Could you check a few things on this model? Use its own coordinates, in mm. A direction names the side the tool comes from. Round coordinates to 2 decimals unless told otherwise and drop trailing zeros. Loops run counter-clockwise (first coordinate to the right, second up) from the corner with the lowest first, then second, coordinate; pieces in that order, holes last.
from build123d import *
from build123d.topology import SkipClean

# Parameters (mm, degrees)
BOSS_EXTRUDE1_DEPTH         = 31.75
BOSS_EXTRUDE4_DEPTH         = 38.1
SKETCH11_R                  = 12.7
BOSS_EXTRUDE5_DEPTH         = 19.05
F_1_4_20_TAPPED_HOLE3_D     = 5.1054
F_1_4_20_TAPPED_HOLE3_DEPTH = 38.1
F_1_4_20_TAPPED_HOLE3_TIP   = 1.533816902
F_1_4_20_TAPPED_HOLE4_D     = 5.1054
F_1_4_20_TAPPED_HOLE4_DEPTH = 11.43
F_1_4_20_TAPPED_HOLE4_TIP   = 1.533816902
CUT_EXTRUDE3_DEPTH          = 3.175
SKETCH17_R                  = 15.875
CUT_EXTRUDE4_DEPTH          = 15.875
FILLET3_R                   = 1.5875
CUT_EXTRUDE5_DEPTH          = 6.35
FILLET4_R                   = 1.5875


with BuildPart() as part:
    # Sketch1 → Boss-Extrude1 (new body)
    with BuildSketch(Plane.XY):
        with BuildLine():
            Line((18.072416828, 26.104602085), (30.120694713, -10.040231571))
            Line((30.120694713, -10.040231571), (6.024138943, -18.072416828))
            ThreePointArc((6.024138943, -18.072416828), (-18.072416828, -6.024138943), (-6.024138943, 18.072416828))
            Line((-6.024138943, 18.072416828), (18.072416828, 26.104602085))
        make_face()
    extrude(amount=BOSS_EXTRUDE1_DEPTH)

    # Sketch10 → Boss-Extrude4 (add)
    with BuildSketch(Plane(origin=(-6.024138943, 18.072416828, 0), x_dir=(0.9486832980505138, 0.31622776601683816, 0), z_dir=(-0.31622776601683816, 0.9486832980505138, 0))):
        Polygon((25.4, 0), (31.75, 0), (40.015050599, -37.192726958), (27.240344607, -40.031550568), (25.4, -31.75), align=None)
    extrude(amount=-BOSS_EXTRUDE4_DEPTH)

    # Sketch11 → Boss-Extrude5 (add)
    with BuildSketch(Plane.XY.offset(31.75)):
        with Locations(Location((0, 0, 0), (0, 0, 180))):
            Circle(SKETCH11_R)
    extrude(amount=BOSS_EXTRUDE5_DEPTH)

    # 1/4-20 Tapped Hole3
    with Locations(Plane.XY.offset(50.8)):
        with Locations((0, 0)):
            Hole(F_1_4_20_TAPPED_HOLE3_D / 2, depth=F_1_4_20_TAPPED_HOLE3_DEPTH)
            with Locations((0, 0, -(F_1_4_20_TAPPED_HOLE3_DEPTH + F_1_4_20_TAPPED_HOLE3_TIP / 2))):  # 118° drill point
                Cone(0, F_1_4_20_TAPPED_HOLE3_D / 2, F_1_4_20_TAPPED_HOLE3_TIP, mode=Mode.SUBTRACT)

    # 1/4-20 Tapped Hole4
    with Locations(Plane(origin=(28.703250202, 9.567750067, -6.723529533), x_dir=(-0.2057983060639255, -0.06859943535464187, -0.9761870592720655), z_dir=(0.9260923589044555, 0.30869745296815215, -0.21693046192214882))):
        with Locations((-38.637542166, 12.7), (-16.412542166, 6.35), (-16.412542166, -6.35), (-38.637542166, -12.7)):
            Hole(F_1_4_20_TAPPED_HOLE4_D / 2, depth=F_1_4_20_TAPPED_HOLE4_DEPTH)
            with Locations((0, 0, -(F_1_4_20_TAPPED_HOLE4_DEPTH + F_1_4_20_TAPPED_HOLE4_TIP / 2))):  # 118° drill point
                Cone(0, F_1_4_20_TAPPED_HOLE4_D / 2, F_1_4_20_TAPPED_HOLE4_TIP, mode=Mode.SUBTRACT)

    # Sketch16 → Cut-Extrude3 (cut)
    with BuildSketch(Plane(origin=(0, 0, 0), x_dir=(-1, 0, 0), z_dir=(0, 0, -1))):
        with BuildLine():
            Line((-30.578183366, -6.540991497), (-16.999386581, -3.994967099))
            ThreePointArc((-16.999386581, -3.994967099), (-15.110000404, -8.753673173), (-11.921633961, -12.759841298))
            Line((-11.921633961, -12.759841298), (-30.578183366, -6.540991497))
        make_face()
        with BuildLine():
            Line((-31.84160072, -5.162718019), (-17.29194463, -2.434657503))
            ThreePointArc((-17.29194463, -2.434657503), (-16.566382092, 5.522127364), (-12.372761203, 12.32289278))
            Line((-12.372761203, 12.32289278), (-22.375649764, 23.235134847))
            Line((-22.375649764, 23.235134847), (-31.84160072, -5.162718019))
        make_face()
        with BuildLine():
            Line((-1.88140239, 17.360853415), (-20.537951794, 23.579703217))
            Line((-20.537951794, 23.579703217), (-11.202529005, 13.395605628))
            ThreePointArc((-11.202529005, 13.395605628), (-6.83579642, 16.068938781), (-1.88140239, 17.360853415))
        make_face()
    extrude(amount=-CUT_EXTRUDE3_DEPTH, mode=Mode.SUBTRACT)

    # Sketch17 → Cut-Extrude4 (cut)
    with BuildSketch(Plane(origin=(0, 0, 0), x_dir=(-1, 0, 0), z_dir=(0, 0, -1))):
        Circle(SKETCH17_R)
    extrude(amount=-CUT_EXTRUDE4_DEPTH, mode=Mode.SUBTRACT)

    # Fillet3
    fillet3_edges = [part.edges().sort_by_distance(p)[0] for p in [
        (31.84160072, -5.162718019, 1.5875),
        (22.375649764, 23.235134847, 1.5875),
        (12.372761203, 12.32289278, 1.5875),
        (17.29194463, -2.434657503, 1.5875),
        (11.202529005, 13.395605628, 1.5875),
        (20.537951794, 23.579703217, 1.5875),
        (1.88140239, 17.360853415, 1.5875),
        (16.999386581, -3.994967099, 1.5875),
        (11.921633961, -12.759841298, 1.5875),
        (30.578183366, -6.540991497, 1.5875),
    ]]
    fillet(fillet3_edges, radius=FILLET3_R)

    # Sketch19 → Cut-Extrude5 (cut)
    with SkipClean():  # the faces are left unmerged after this step: merging them gives an invalid solid
        with BuildSketch(Plane(origin=(0, 0, 15.875), x_dir=(-1, 0, 0), z_dir=(0, 0, -1))):
            with BuildLine():
                Line((1.5875, 4.490128061), (1.5875, 15.795425564))
                ThreePointArc((1.5875, 15.795425564), (9.33109088, 12.843144786), (14.531777932, 6.390857152))
                Line((14.531777932, 6.390857152), (3.779801072, 2.897328097))
                ThreePointArc((3.779801072, 2.897328097), (2.799327264, 3.852943436), (1.5875, 4.490128061))
            make_face()
            with BuildLine():
                Line((-1.5875, 4.490128061), (-1.5875, 15.795425564))
                ThreePointArc((-1.5875, 15.795425564), (-9.33109088, 12.843144786), (-14.531777932, 6.390857152))
                Line((-14.531777932, 6.390857152), (-3.779801072, 2.897328097))
                ThreePointArc((-3.779801072, 2.897328097), (-2.799327264, 3.852943436), (-1.5875, 4.490128061))
            make_face()
            with BuildLine():
                Line((4.76093003, -0.122276342), (15.512906889, 3.371252713))
                ThreePointArc((15.512906889, 3.371252713), (15.098022196, -4.905644786), (10.568632679, -11.845658627))
                Line((10.568632679, -11.845658627), (3.923545533, -2.69948082))
                ThreePointArc((3.923545533, -2.69948082), (4.529406659, -1.471693436), (4.76093003, -0.122276342))
            make_face()
            with BuildLine():
                Line((1.354916576, -4.565698996), (8.000003722, -13.711876803))
                ThreePointArc((8.000003722, -13.711876803), (0, -15.875), (-8.000003722, -13.711876803))
                Line((-8.000003722, -13.711876803), (-1.354916576, -4.565698996))
                ThreePointArc((-1.354916576, -4.565698996), (0, -4.7625), (1.354916576, -4.565698996))
            make_face()
            with BuildLine():
                Line((-3.923545533, -2.69948082), (-10.568632679, -11.845658627))
                ThreePointArc((-10.568632679, -11.845658627), (-15.098022196, -4.905644786), (-15.512906889, 3.371252713))
                Line((-15.512906889, 3.371252713), (-4.76093003, -0.122276342))
                ThreePointArc((-4.76093003, -0.122276342), (-4.529406659, -1.471693436), (-3.923545533, -2.69948082))
            make_face()
        extrude(amount=-CUT_EXTRUDE5_DEPTH, mode=Mode.SUBTRACT)

    # Fillet4
    # the kernel refuses this fillet: 1.5875 mm, written as the material it adds along each edge
    with BuildSketch(Plane(origin=(-3.779801072, 2.897328097, 15.875), x_dir=(0.678616300980504, 0.7344929652784552, 0), z_dir=(0, 0, 1)), Plane(origin=(1.5875, 4.490128061, 15.875), x_dir=(0.9082482904638647, -0.4184316465917308, 0), z_dir=(0, 0, 1)), Plane(origin=(1.354916576, -4.565698996, 15.875), x_dir=(-0.9807362530563359, -0.1953366374775062, 0), z_dir=(0, 0, 1)), Plane(origin=(4.76093003, -0.122276342, 15.875), x_dir=(-0.1172879872498498, -0.9930979448407287, 0), z_dir=(0, 0, 1))) as fillet4_piece_1:
        with BuildLine():
            CenterArc((1.019590872, 1.580803791), FILLET4_R, 204.735610317, 60)
            Line((-0.422253289, 0.916543552), (0, 0))
            ThreePointArc((0, 0), (0.436967517, 0.020088626), (0.873935033, 0))
        make_face()
    extrude(amount=8.872833134)
    with BuildSketch(Plane(origin=(-1.5875, 4.490128061, 15.875), x_dir=(0, 1, 0), z_dir=(0, 0, 1)), Plane(origin=(3.779801072, 2.897328097, 15.875), x_dir=(0.9510565162951539, 0.30901699437494645, 0), z_dir=(0, 0, 1)), Plane(origin=(-4.76093003, -0.122276342, 15.875), x_dir=(-0.9510565162951536, 0.3090169943749475, 0), z_dir=(0, 0, 1)), Plane(origin=(-1.354916576, -4.565698996, 15.875), x_dir=(-0.5877852522924731, -0.8090169943749473, 0), z_dir=(0, 0, 1)), Plane(origin=(3.923545533, -2.69948082, 15.875), x_dir=(0.5877852522924732, -0.8090169943749472, 0), z_dir=(0, 0, 1))) as fillet4_piece_2:
        with BuildLine():
            CenterArc((1.009133253, 1.5875), FILLET4_R, 210, 60)
            ThreePointArc((-0.365682075, 0.79375), (-0.164595577, 0.405280717), (0, 0))
            Line((0, 0), (1.009133253, 0))
        make_face()
    extrude(amount=8.872833134)
    with BuildSketch(Plane(origin=(-1.5875, 15.795425564, 15.875), x_dir=(-0.9868856549354627, -0.16142089109716581, 0), z_dir=(0, 0, 1)), Plane(origin=(14.531777932, 6.390857152, 15.875), x_dir=(-0.4584848292240369, 0.8887022343684108, 0), z_dir=(0, 0, 1)), Plane(origin=(-15.512906889, 3.371252713, 15.875), x_dir=(-0.15144404853577972, -0.9884658315607537, 0), z_dir=(0, 0, 1)), Plane(origin=(-8.000003722, -13.711876803, 15.875), x_dir=(0.8932880855464623, -0.4494845895253098, 0), z_dir=(0, 0, 1)), Plane(origin=(10.568632679, -11.845658627, 15.875), x_dir=(0.7035264471488165, 0.7106690778148178, 0), z_dir=(0, 0, 1))) as fillet4_piece_3:
        with BuildLine():
            CenterArc((1.867758316, 1.584453457), FILLET4_R, 170.710620558, 102.839588407)
            Line((0.301077339, 1.840709121), (0, 0))
            ThreePointArc((0, 0), (0.983030693, -0.030465433), (1.966061385, 0))
        make_face()
    extrude(amount=11.265153463)
    with BuildSketch(Plane(origin=(-14.531777932, 6.390857152, 15.875), x_dir=(0.45848482922403855, 0.88870223436841, 0), z_dir=(0, 0, 1)), Plane(origin=(1.5875, 15.795425564, 15.875), x_dir=(0.9868856549354627, -0.16142089109716573, 0), z_dir=(0, 0, 1)), Plane(origin=(-10.568632679, -11.845658627, 15.875), x_dir=(-0.7035264471488155, 0.7106690778148187, 0), z_dir=(0, 0, 1)), Plane(origin=(8.000003722, -13.711876803, 15.875), x_dir=(-0.8932880855464624, -0.4494845895253094, 0), z_dir=(0, 0, 1)), Plane(origin=(15.512906889, 3.371252713, 15.875), x_dir=(0.1514440485357779, -0.988465831560754, 0), z_dir=(0, 0, 1))) as fillet4_piece_4:
        with BuildLine():
            CenterArc((1.867758316, -1.584453457), FILLET4_R, 86.449791035, 102.839588407)
            Line((0.301077339, -1.840709121), (0, 0))
            ThreePointArc((0, 0), (0.983030693, 0.030465433), (1.966061385, 0))
        make_face()
    extrude(amount=11.265153463)
    with BuildSketch(Plane(origin=(-3.923545533, -2.69948082, 15.875), x_dir=(-0.5877852522924727, -0.8090169943749477, 0), z_dir=(0, 0, 1))) as fillet4_piece_5:
        with BuildLine():
            CenterArc((1.009133253, -1.5875), FILLET4_R, 90, 60)
            ThreePointArc((-0.365682075, -0.79375), (-0.164595577, -0.405280717), (0, 0))
            Line((0, 0), (1.009133253, 0))
        make_face()
    extrude(amount=8.872833134)


solid = part.part
Item 1: If we section it at B-B, the plane x = -11: Please give me the cut outline in (y, z) (3 decimals).
Results list:
outline: (-15.553, 0) - (-11.446, 0) - (-11.446, 15.875) - (-10.972, 15.875) - (-10.972, 22.225) - (1.905, 22.225) - (1.905, 15.875) - (5.243, 15.875) - (5.243, 22.225) - (11.446, 22.225) - (11.446, 0) - (15.553, 0) - (15.553, 31.75) - (6.347, 31.75) - (6.347, 50.8) - (-6.347, 50.8) - (-6.347, 31.75) - (-15.553, 31.75) - close
Item 2: Will these pins go through, and if not, where does the flat tip stop? pin 1 (6 mm diameter, centred on x = 21.5, y = -4.5, fed in from +Z); pin 2 (10 mm diameter, centred on y = 7.5, z = 23, fed in from +X); pin 3 (5 mm diameter, centred on y = 9, z = 20, fed in from -X).
Results list:
pin 1: stops at z = 31.75
pin 2: stops at x = 38.39
pin 3: stops at x = -17.91
Item 3: If I drill on line 1 along Y through (x, z) = (0, 34); line 2 along X through (y, z) = (0, 6.75) (3 decimals); line 3 along Z through (x, y) = (-12.5, 7.5) (3 decimals), over which ranges is the centre line in solid material (lowest first)?
Results list:
line 1: y = -12.7 to -2.55, 2.55 to 12.7
line 2: x = -19.05 to -15.875, 15.875 to 35.049
line 3: z = 22.225 to 31.75
Item 4: If we section it at A-A, the plane z = 41: Please give me the cut outline in (x, y).
Results list:
outline: circle Ø25.4 at (0, 0); hole circle Ø5.11 at (0, 0)
Item 5: For faces 1 (the flat face through (24.897, 8.58, 35.949)), 2 (the flat face through (27.054, 9.199, 1.565)), which set-ups out of +Z, -Z, +X, -X, +Y, -Y let a thin tool reach every point of the face, with its end or its side?
Results list:
face 1: +Z, -Y
face 2: -Z
Item 6: We'd pull the mould along X, two halves only. Please class faces 3 (the cylindrical face through (22.08, 21.72, 1.61)), 4 (the cylindrical face through (-2, 15, 19)): released by +X, released by -X, zero draft, split by the parting line, or undercut.
Results list:
face 3: undercut
face 4: undercut
